Can you work these out from the drawing? Everything is in mm from the part's minimum corner. Coordinates: 2 decimals unless noted, no trailing zeros. Order: outer loops, then holes, each group sorted by start corner. A loop starts at its lowest first (then second) coordinate and runs counter-clockwise, first axis right, second up. Notation, with made-up numbers: (55.5, 75.5) -> (101.5, 75.5) arc R15 ccw to (101.5, 91.5) -> close; hole circle Ø7 at (23.5, 83). An arc over 180 degrees is marked (long way). Return JSON: item names as keys, results as strings. Group by question number.
1) If we section it at B-B, the plane y = 4: Please give me the cut outline in (x, z), then the cut area to 3 significant figures.
2) If we section it at C-C, the plane z = 3.9: Please give me the cut outline in (x, y), then the cut area to 3 significant figures.
3) If we section it at A-A, the plane x = 48.75: Please give me the cut outline in (y, z), then the cut area to 3 significant figures.
4) For pin 1 (2.5 mm diameter, centred on x = 17, y = 4, fed in from -Z), with a flat end and sliding along its axis, tell me the tip position at first contact or that it passes through.
5) If I drill on probe 1 along Y at (x, z) = (3, 2.75); probe 2 along X at (y, z) = (3.5, 2.05); probe 3 along Y at (x, z) = (33, 1.7), over which ranges is the centre line in solid material (lowest first)? Write a range as from..to.
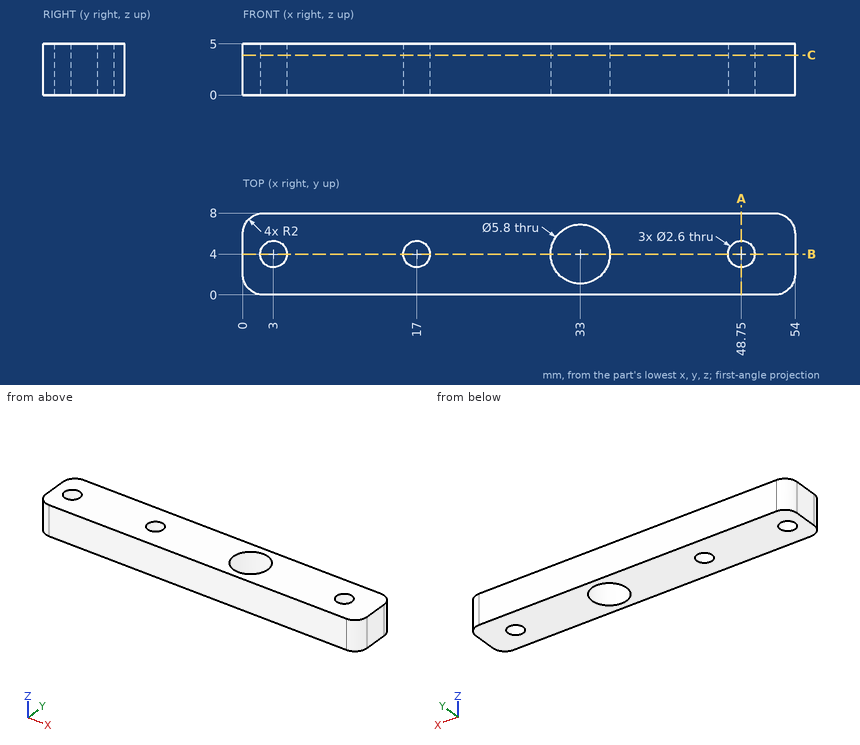
Result sheet:
{
 "1": {"outline": "(0, 0) -> (1.7, 0) -> (1.7, 5) -> (0, 5) -> close; (4.3, 0) -> (15.7, 0) -> (15.7, 5) -> (4.3, 5) -> close; (18.3, 0) -> (30.1, 0) -> (30.1, 5) -> (18.3, 5) -> close; (35.9, 0) -> (47.45, 0) -> (47.45, 5) -> (35.9, 5) -> close; (50.05, 0) -> (54, 0) -> (54, 5) -> (50.05, 5) -> close", "area": "202 mm2"},
 "2": {"outline": "(0, 2) arc R2 ccw to (2, 0) -> (52, 0) arc R2 ccw to (54, 2) -> (54, 6) arc R2 ccw to (52, 8) -> (2, 8) arc R2 ccw to (0, 6) -> close; hole circle Ø2.6 at (3, 4); hole circle Ø2.6 at (17, 4); hole circle Ø5.8 at (33, 4); hole circle Ø2.6 at (48.75, 4)", "area": "386 mm2"},
 "3": {"outline": "(0, 0) -> (2.7, 0) -> (2.7, 5) -> (0, 5) -> close; (5.3, 0) -> (8, 0) -> (8, 5) -> (5.3, 5) -> close", "area": "27.0 mm2"},
 "4": {"pin 1": "passes through"},
 "5": {"probe 1": "y = 0..2.7, 5.3..8", "probe 2": "x = 0..1.8, 4.2..15.8, 18.2..30.14, 35.86..47.55, 49.95..54", "probe 3": "y = 0..1.1, 6.9..8"}
}
